Source: CAD feature listing. Evaluate the final solid. Frame: model axes, mm. Face numbers are marked on the shaded views. A direction names the side the tool comes from. Coordinates: 2 decimals unless noted, no trailing zeros. Loops run counter-clockwise (first coordinate to the right, second up) from the corner with the lowest first, then second, coordinate; pieces in that order, holes last. Notation, with made-up numbers: (-2, 48) -> (19, 48) arc R21 ccw to (19, 72) -> close; hole circle Ø7 at (-8.5, 5). An arc over 180 degrees is marked (long way). Answer as CSV lines item,"result".
from build123d import *

# Parameters (mm, degrees)
F0_W     = 110
F0_H     = 300
F1_DEPTH = 240
F3_DEPTH = 110
F4_R     = 50
F4_R_2   = 25
F5_DEPTH = 410.001
F6_R     = 130
F7_R     = 50
F8_R     = 20


with BuildPart() as f1:
    # F0 (on Front) → F1 (new body, symmetric)
    with BuildSketch(Plane.XZ):
        with BuildLine():
            Line((154.9193338483, 110), (279.1057147391, 110))
            ThreePointArc((279.1057147391, 110), (0, 300), (-279.1057147391, 110))
            Line((-279.1057147391, 110), (-154.9193338483, 110))
            ThreePointArc((-154.9193338483, 110), (0, 190), (154.9193338483, 110))
        make_face()
        with BuildLine():
            Line((190, 0), (300, 0))
            ThreePointArc((300, 0), (294.7301430306, 55.9834153044), (279.1057147391, 110))
            Line((279.1057147391, 110), (154.9193338483, 110))
            ThreePointArc((154.9193338483, 110), (181.0175038928, 57.7292238334), (190, 0))
        make_face()
        with BuildLine():
            Line((-560, 0), (-300, 0))
            ThreePointArc((-300, 0), (-294.7301430306, 55.9834153044), (-279.1057147391, 110))
            Line((-279.1057147391, 110), (-560, 110))
            Line((-560, 110), (-560, 0))
        make_face()
        with BuildLine():
            ThreePointArc((-279.1057147391, 110), (-294.7301430306, 55.9834153044), (-300, 0))
            Line((-300, 0), (-190, 0))
            ThreePointArc((-190, 0), (-181.0175038928, 57.7292238334), (-154.9193338483, 110))
            Line((-154.9193338483, 110), (-279.1057147391, 110))
        make_face()
        with BuildLine():
            ThreePointArc((279.1057147391, 110), (294.7301430306, 55.9834153044), (300, 0))
            Line((300, 0), (510, 0))
            Line((510, 0), (510, 110))
            Line((510, 110), (400, 110))
            Line((400, 110), (279.1057147391, 110))
        make_face()
        with Locations((455, 260)):
            Rectangle(F0_W, F0_H)
    extrude(amount=F1_DEPTH, both=True)

    # F2 (on face) → F3 (cut, through all)
    with BuildSketch(Plane.YZ.offset(510)):
        with BuildLine():
            ThreePointArc((-65, 250), (0, 185), (65, 250))
            ThreePointArc((65, 250), (0, 315), (-65, 250))
        make_face()
        with BuildLine():
            ThreePointArc((-65, 250), (0, 315), (65, 250))
            Line((65, 250), (65, 410))
            Line((65, 410), (-65, 410))
            Line((-65, 410), (-65, 250))
        make_face()
    extrude(amount=-F3_DEPTH, mode=Mode.SUBTRACT)

    # F4 (on Top) → F5 (cut, through all)
    with BuildSketch(Plane.XY):
        with Locations((-419.5528573695, 110)):
            Circle(F4_R)
        with Locations((-419.5528573695, -110)):
            Circle(F4_R)
        Circle(F4_R_2)
    extrude(amount=F5_DEPTH, mode=Mode.SUBTRACT)

    # F6
    f6_edges = [f1.edges().sort_by_distance(p)[0] for p in [
        (-560, 240, 55),
        (-560, -240, 55),
    ]]
    fillet(f6_edges, radius=F6_R)

    # F7
    f7_edges = [f1.edges().sort_by_distance(p)[0] for p in [
        (455, 240, 410),
        (455, -240, 410),
    ]]
    fillet(f7_edges, radius=F7_R)

    # F8
    f8_edges = [f1.edges().sort_by_distance(p)[0] for p in [
        (-279.105715, 0, 110),
        (279.105715, 0, 110),
    ]]
    fillet(f8_edges, radius=F8_R)


solid = f1.part
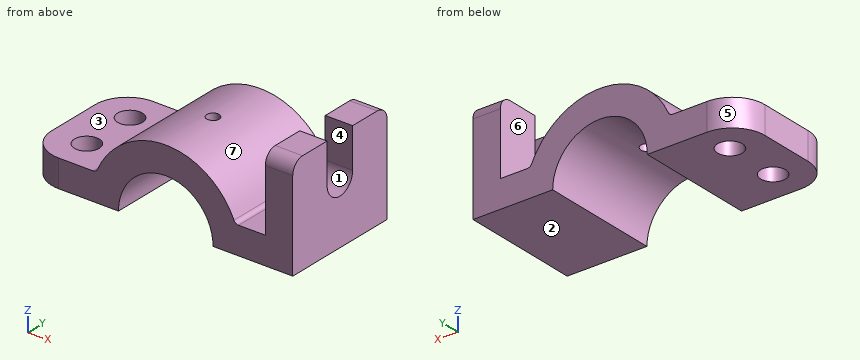
(1) Cut plane C-C (y = 0). Return the cut outline in (x, z) (3 decimals).
Computed values:
outline,"(-560, 0) -> (-190, 0) arc R190 cw to (-25, 188.348) -> (-25, 298.957) arc R300 ccw to (-274.129, 121.875) arc R20 cw to (-292.404, 110) -> (-560, 110) -> close; (25, 188.348) arc R190 cw to (190, 0) -> (510, 0) -> (510, 185) -> (400, 185) -> (400, 110) -> (292.404, 110) arc R20 cw to (274.129, 121.875) arc R300 ccw to (25, 298.957) -> close"
(2) Draft query along X for the marked faces 4, 5, 6 and 7. Return one class per face: released by +X, released by -X, zero draft, split by the parting line, or undercut.
Computed values:
face 4,"zero draft"
face 5,"released by -X"
face 6,"undercut"
face 7,"undercut"
(3) Access query for the marked faces 1, 2 and 3. Directions: +Z, -Z, +X, -X, +Y, -Y. A direction counts if a zero-diameter tool reaches every point of the face in a straight line with its end or side. Return the directions, or none.
Computed values:
face 1,"+Z, +X"
face 2,"-Z, +X, -X, +Y, -Y"
face 3,"+Z, -X, +Y, -Y"
(4) Cut plane D-D (z = 58). Return the cut outline in (x, y).
Computed values:
outline,"(-560, -110) arc R130 ccw to (-430, -240) -> (-180.93, -240) -> (-180.93, 240) -> (-430, 240) arc R130 ccw to (-560, 110) -> close; (180.93, -240) -> (510, -240) -> (510, 240) -> (180.93, 240) -> close; hole circle Ø100 at (-419.55, -110); hole circle Ø100 at (-419.55, 110)"
(5) Cut plane B-B (x = 0). Return the cut outline in (y, z), then the cut area to 3 significant figures.
Computed values:
outline,"(-240, 190) -> (-25, 190) -> (-25, 300) -> (-240, 300) -> close; (25, 190) -> (240, 190) -> (240, 300) -> (25, 300) -> close"
area,"47,300 mm^2"
(6) Cut plane A-A (z = 219.5). Return the cut outline in (x, y), then the cut area to 3 significant figures.
Computed values:
outline,"(-204.5, -240) -> (204.5, -240) -> (204.5, 240) -> (-204.5, 240) -> close; (400, -240) -> (510, -240) -> (510, -57.4) -> (400, -57.4) -> close; (400, 57.4) -> (510, 57.4) -> (510, 240) -> (400, 240) -> close; hole circle Ø50 at (0, 0)"
area,"235,000 mm^2"
(7) Material intervals for L1, parallel to Y at x = 0, z = 245; L2, parallel to X at y = -110, z = 74.5; L3, parallel to X at y = 121.5, z = 35, sorted ascending. Write a range as [from, to].
Computed values:
L1,"[-240, -25], [25, 240]"
L2,"[-560, -469.55], [-369.55, -174.78], [174.78, 510]"
L3,"[-559.49, -468.21], [-370.89, -186.75], [186.75, 510]"
(8) Pin query (flat end, axial travel): pin 1 Ø3 at (x, y) = (129.5, 129.5) entering from +Z; pin 2 Ø2 at (y, z) = (176.5, 336) entering from -X; pin 3 Ø12 at (x, y) = (-81.5, 139.5) entering from +Z. Return the tip coordinate at first contact, or that it passes through.
Computed values:
pin 1,"z = 271.32"
pin 2,"x = 400"
pin 3,"z = 290.34"
